```python
from build123d import *

# Parameters (mm, degrees)
F0_R     = 73
F1_DEPTH = 86
F5_W     = 254
F5_H     = 104
F6_DEPTH = 17


with BuildPart() as f1:
    # F0 (on Front) → F1 (new body)
    with BuildSketch(Plane.XZ):
        with Locations((0, 86)):
            Circle(F0_R)
    extrude(amount=-F1_DEPTH)

    # F3 (on offset) → F4 (revolve)
    with BuildSketch(Plane.XZ.offset(-52)):
        Polygon((98, 164), (60, 164), (60, 17), (109.011107, 17), (94, 43), (94, 127), (98, 133.928203), align=None)
    revolve(axis=Axis((60, 52, 90.5), (0, 0, 1)))

    # F5 (on Top) → F6 (join)
    with BuildSketch(Plane.XY):
        with Locations((0, 52)):
            Rectangle(F5_W, F5_H)
    extrude(amount=F6_DEPTH)


solid = f1.part
```
Geometry: final body of the model. Coordinates: model frame, mm. A direction names the side the tool comes from. Coordinates: 2 decimals unless noted, no trailing zeros. Loops run counter-clockwise (first coordinate to the right, second up) from the corner with the lowest first, then second, coordinate; pieces in that order, holes last. Notation, with made-up numbers: (63, 19.25) -> (87, 19.25) arc R21 ccw to (87, 37.25) -> close; hole circle Ø5 at (-8, 6). An arc over 180 degrees is marked (long way). Use a Markdown table: item, result. Add a question column.
(1) Mould query, pull axis Z, two halves, no side actions, for faces 1 (the flat face through (59, 53, 164)), 2 (the cylindrical face through (-68.277, 42.398, 111.83)), 3 (the flat face through (-2, 104, 8)). Classes: pulls with the +Z half, pulls with the -Z half, needs draft (parallel to the pull), parting line crosses it, or undercut.
(2) Section query B-B, the plane y = 52. Return loops of the section in (x, z).
(3) Section query D-D, the plane z = 22. Return loops of the section in (x, y).
(4) Pin query (flat end, axial travel): pin 1 Ø1.5 at (y, z) = (57, 115) entering from +X; pin 2 Ø1 at (y, z) = (46.5, 110) entering from +X; pin 3 Ø5 at (x, z) = (63.5, 48) entering from +Y. Return the tip coordinate at first contact, or that it passes through.
(5) Access query for faces 4 (the flat face through (-1, 86, 89)), 5 (the flat face through (-2, 0, 78)), 6 (the conical face through (96.376, 50.777, 38.849)), 7 (the cylindrical face through (96.245, 63.414, 152.516)), 8 (the flat face through (-2, 53, 0)). Directions: +Z, -Z, +X, -X, +Y, -Y. A direction counts if a zero-diameter tool reaches every point of the face in a straight line with its end or side. Return the directions, or none.
(6) Line query: line 1 along Y through (x, z) = (-37, 92.5); line 2 along Z through (x, y) = (25, 98.5); line 3 along Z through (x, y) = (-2, 71.5). Output: solid intervals per line, ascending.
(7) Section query C-C, the plane z = 86. Return loops of the section in (x, y), plus the area to 3 significant figures.
(8) Section query A-A, the plane x = 0. Return loops of the section in (y, z), plus the area to 3 significant figures.
Answer:
| question | item | result |
|---|---|---|
| 1 | face 1 | pulls with the +Z half |
| 1 | face 2 | undercut |
| 1 | face 3 | needs draft |
| 2 | outline | (-127, 0) -> (127, 0) -> (127, 17) -> (109.01, 17) -> (94, 43) -> (94, 127) -> (98, 133.93) -> (98, 164) -> (22, 164) -> (22, 155.61) arc R73 ccw to (-23.83, 17) -> (-127, 17) -> close |
| 3 | outline | (-35.11, 0) -> (35.11, 0) -> (35.11, 13.17) arc R46.12 ccw (long way) to (28.83, 86) -> (-35.11, 86) -> close |
| 4 | pin 1 | stops at x = 93.73 |
| 4 | pin 2 | stops at x = 93.63 |
| 4 | pin 3 | stops at y = 86 |
| 5 | face 4 | -X, +Y |
| 5 | face 5 | +Z, -Z, +X, -X, -Y |
| 5 | face 6 | none |
| 5 | face 7 | +Z |
| 5 | face 8 | -Z, +X, -X, +Y, -Y |
| 6 | line 1 | y = 0 to 86 |
| 6 | line 2 | z = 0 to 17 |
| 6 | line 3 | z = 0 to 158.97 |
| 7 | outline | (-73, 0) -> (73, 0) -> (73, 20.58) arc R34 ccw to (73, 83.42) -> (73, 86) -> (-73, 86) -> close |
| 7 | area | 13,500 mm^2 |
| 8 | outline | (0, 0) -> (104, 0) -> (104, 17) -> (86, 17) -> (86, 159) -> (0, 159) -> close |
| 8 | area | 14,000 mm^2 |
